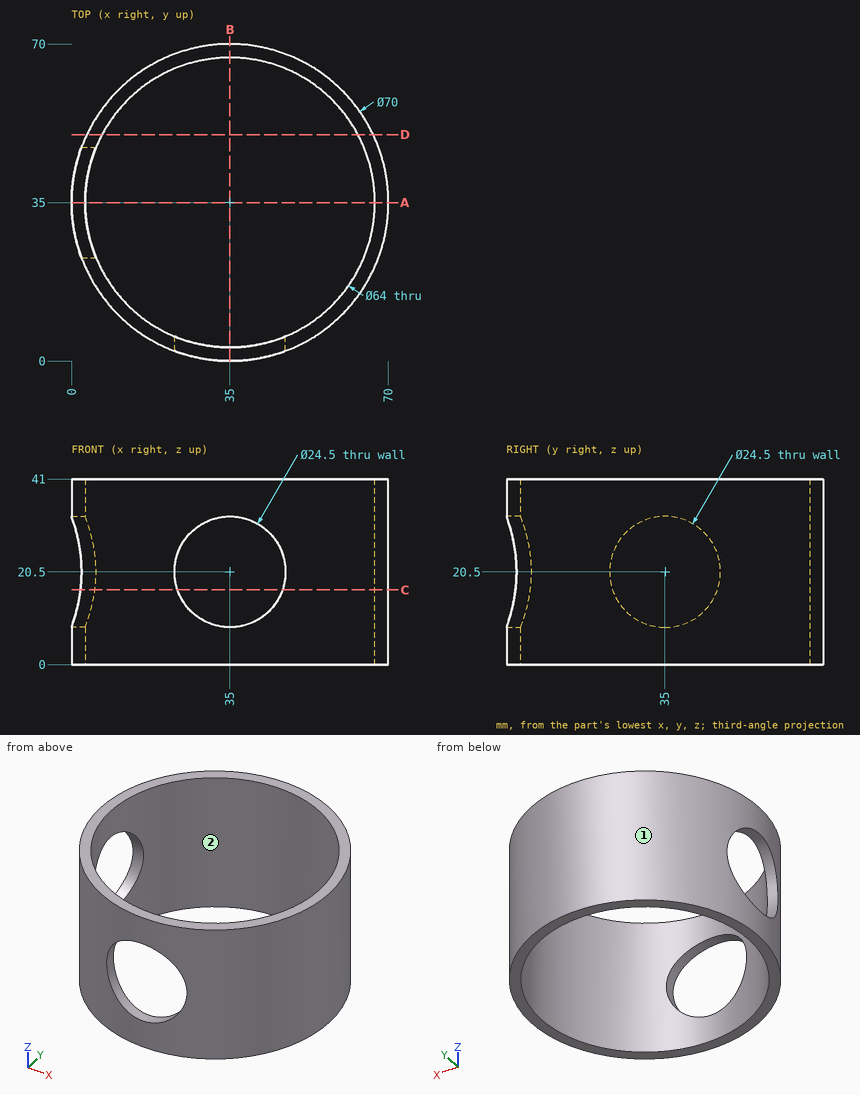
The figure shows three views and two pictorial views of one solid part (mm, origin at its lowest corner). Answer the questions. Round coordinates to 2 decimals unless told otherwise and drop trailing zeros. Loops run counter-clockwise (first coordinate to the right, second up) from the corner with the lowest first, then second, coordinate; pieces in that order, holes last. Notation, with made-up numbers: (-6, -40) - (22, -40) arc R17 ccw to (22, -21) - close; hole circle Ø1 at (33.5, -27). An arc over 180 degrees is marked (long way). Use one line per item in the form item = value. Start each with the question number.
(1) Consider line 1 (Y direction, x = 36, z = 7); line 2 (Y direction, x = 35, z = 21.5); line 3 (X direction, y = 7, z = 23). Determine where each line is inside the solid, lowest interval first.
(2) Determine the mould class of the marked faces 1 and 2 for opening direction X: +X half, -X half, draft (parallel to the pull), parting line (faces both ways), or undercut.
(3) Find section C-C on z = 16.5. Determine the outline of the cut face in (x, y).
(4) Find section A-A on y = 35. Determine the outline of the cut face in (x, z), and give its area (4 significant figures).
(5) Find section D-D on y = 50. Determine the outline of the cut face in (x, z).
(6) Flat-ended cylindrical pins translate along their axes: P1, Ø8, axis at y = 19.5, z = 6.5, coming from the +X side; P2, Ø3, axis at y = 15, z = 4, coming from the +X side; P3, Ø4, axis at x = 47.5, z = 5, coming from the +Y side. Find the tip coordinate at first contact, or state that the pin passes through.
Answer list:
q1.line_1 = 0.01 to 3.02, 66.98 to 69.99
q1.line_2 = 67 to 70
q1.line_3 = 14 to 19.51, 50.49 to 56
q2.face_1 = parting line
q2.face_2 = undercut
q3.outline = (1.97, 23.42) arc R35 ccw to (23.42, 1.97) - (23.42, 5.17) arc R32 cw to (5.17, 23.42) - close; (1.97, 46.58) - (5.17, 46.58) arc R32 cw (long way) to (46.58, 5.17) - (46.58, 1.97) arc R35 ccw (long way) to start
q4.outline = (0, 0) - (3, 0) - (3, 8.25) - (0, 8.25) - close; (0, 32.75) - (3, 32.75) - (3, 41) - (0, 41) - close; (67, 0) - (70, 0) - (70, 41) - (67, 41) - close
q4.area = 172.5 mm^2
q5.outline = (3.38, 0) - (6.73, 0) - (6.73, 41) - (3.38, 41) - close; (63.27, 0) - (66.62, 0) - (66.62, 41) - (63.27, 41) - close
q6.P1 = 68.06
q6.P2 = 64.71
q6.P3 = 68.39
